For this review, use the dimensioned drawing (mm, ordinates from the lowest corner) and the shaded views. A direction names the side the tool comes from. Coordinates: 2 decimals unless noted, no trailing zeros. Write each loop counter-clockwise with the first axis right and the second up, starting at its lowest first coordinate (ties: lowest second). Pieces come first, ordered by that corner, then holes. Notation, with made-up numbers: M 27.5,56 L 61.5,56 A32 ccw 61.5,89 Z; hole C -25,-20 d7. An arc over 180 degrees is marked long. Return JSON: item names as keys, results as strings. Group by question number.
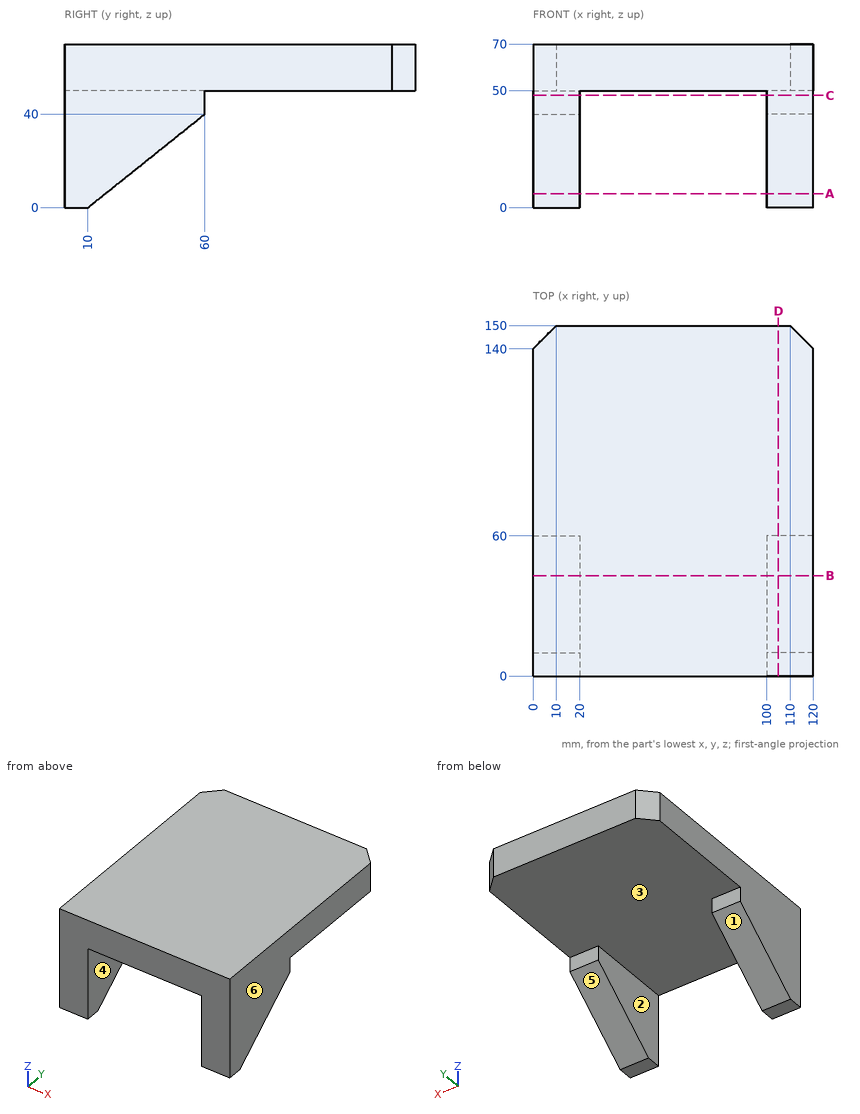
Item 1: Add section D-D (x = 105). Write out the cut boundary in (y, z), plus the area to 3 significant figures.
Item 2: The part is to be moulded in two halves that separate along X. For the marked faces 3, 4, 5 and 6, say which applies: pulls with the +X half, pulls with the -X half, needs draft (parallel to the pull), parting line crosses it, or undercut.
Item 3: Machinability: for the marked faces 1 and 2, which of the approach directions +Z, -Z, +X, -X, +Y, -Y give a long, thin tool a straight path to every point of the face, cutting with its end or side? Answer none if there is none.
Item 4: For line 1 (X direction, y = 38.5, z = 44); line 2 (Y direction, x = 13, z = 49); line 3 (Z direction, x = 41.5, y = 36), list the stretches that pass through material, from the lowest coordinate up.
Item 5: Add section B-B (y = 43). Write out the cut boundary in (x, z), plus the area to 3 significant figures.
Item 6: Add section C-C (z = 48). Write out the cut boundary in (x, y).
Item 7: Add section A-A (z = 6). Write out the cut boundary in (x, y).
Item 8: For pin 1 (2 mm diameter, centred on x = 73, y = 86, fed in from -Z); pin 2 (3 mm diameter, centred on x = 13, z = 43, fed in from +Y), all flat-tipped, find the tip position at first contact; note any pin that passes through.
Geometry check:
{
 "1": {"outline": "M 0,0 L 10,0 L 60,40 L 60,50 L 150,50 L 150,70 L 0,70 Z", "area": "5,000 mm^2"},
 "2": {"face 3": "undercut", "face 4": "undercut", "face 5": "needs draft", "face 6": "pulls with the +X half"},
 "3": {"face 1": "-Z, +X, -X, +Y", "face 2": "-Z, +Y, -Y"},
 "4": {"line 1": "0 to 20, 100 to 120", "line 2": "0 to 60", "line 3": "50 to 70"},
 "5": {"outline": "M 0,26.4 L 20,26.4 L 20,50 L 100,50 L 100,26.4 L 120,26.4 L 120,70 L 0,70 Z", "area": "3,340 mm^2"},
 "6": {"outline": "M 0,0 L 20,0 L 20,60 L 0,60 Z; M 100,0 L 120,0 L 120,60 L 100,60 Z"},
 "7": {"outline": "M 0,0 L 20,0 L 20,17.5 L 0,17.5 Z; M 100,0 L 120,0 L 120,17.5 L 100,17.5 Z"},
 "8": {"pin 1": "z = 50", "pin 2": "y = 60"}
}
